from build123d import *

# Parameters (mm, degrees)
SKETCH1_W           = 20
SKETCH1_H           = 20
SKETCH1_W_2         = 11.2
SKETCH1_H_2         = 11.2
BOSS_EXTRUDE1_DEPTH = 200
SKETCH2_R           = 1.45
CUT_EXTRUDE1_DEPTH  = 202.990098767
FILLET3_SIZE        = 5
FILLET4_SIZE        = 10
SKETCH4_R           = 2.25
CUT_EXTRUDE3_DEPTH  = 202.990098886
FILLET6_R           = 1
SKETCH5_W           = 3
SKETCH5_H           = 20
CUT_EXTRUDE4_DEPTH  = 10
FILLET7_START       = 8.5
FILLET7_DEPTH       = 3
SKETCH7_R           = 0.5
CUT_EXTRUDE6_DEPTH  = 5
SKETCH8_W           = 10
SKETCH8_H           = 2.5
BOSS_EXTRUDE2_DEPTH = 10
FILLET8_R           = 5


with BuildPart() as part:
    # Sketch1 → Boss-Extrude1 (new body)
    with BuildSketch(Plane(origin=(0, 0, 0), x_dir=(1, 0, 0), z_dir=(0, 1, 0))):
        with Locations((10, -10)):
            Rectangle(SKETCH1_W, SKETCH1_H)
        with Locations((10, -10)):
            Rectangle(SKETCH1_W_2, SKETCH1_H_2, mode=Mode.SUBTRACT)
    extrude(amount=BOSS_EXTRUDE1_DEPTH)

    # Sketch2 → Cut-Extrude1 (cut, through all)
    with BuildSketch(Plane.ZY):
        with Locations((8.5, 195)):
            Circle(SKETCH2_R)
    extrude(amount=-CUT_EXTRUDE1_DEPTH, mode=Mode.SUBTRACT)

    # Fillet3
    # a fillet whose section is not a circle: 5 mm, written as the material it adds along each edge
    with BuildSketch(Plane(origin=(4.4, 0, 15.6), x_dir=(1, 0, 0), z_dir=(0, 1, 0))) as fillet3_piece_1:
        with BuildLine():
            Bezier((FILLET3_SIZE, 0), (0, 0), (0, FILLET3_SIZE), weights=[1, 0.052631579, 1])
            Line((0, FILLET3_SIZE), (0, 0))
            Line((0, 0), (FILLET3_SIZE, 0))
        make_face()
    extrude(amount=200)
    with BuildSketch(Plane(origin=(15.6, 0, 15.6), x_dir=(-1, 0, 0), z_dir=(0, 1, 0))) as fillet3_piece_2:
        with BuildLine():
            Bezier((FILLET3_SIZE, 0), (0, 0), (0, -FILLET3_SIZE), weights=[1, 0.052631579, 1])
            Line((0, -FILLET3_SIZE), (0, 0))
            Line((0, 0), (FILLET3_SIZE, 0))
        make_face()
    extrude(amount=200)

    # Fillet4
    # a fillet whose section is not a circle: 10 mm, written as the material it takes off along each edge
    with BuildSketch(Plane(origin=(0, -25, 20), x_dir=(0, 0, -1), z_dir=(0, 1, 0)), Plane(origin=(20, -25, 20), x_dir=(-1, 0, 0), z_dir=(0, 1, 0))) as fillet4_piece_1:
        with BuildLine():
            Bezier((FILLET4_SIZE, 0), (0, 0), (0, -FILLET4_SIZE), weights=[1, 0.052631579, 1])
            Line((0, -FILLET4_SIZE), (0, 0))
            Line((0, 0), (FILLET4_SIZE, 0))
        make_face()
    extrude(amount=250, mode=Mode.SUBTRACT)

    # Sketch4 → Cut-Extrude3 (cut, through all)
    with BuildSketch(Plane(origin=(0, 200, 0), x_dir=(1, 0, 0), z_dir=(0, 1, 0))):
        with Locations((10, -20)):
            Circle(SKETCH4_R)
    extrude(amount=-CUT_EXTRUDE3_DEPTH, mode=Mode.SUBTRACT)

    # Fillet6
    fillet6_edges = [part.edges().sort_by_distance(p)[0] for p in [
        (11.759792875, 100, 18.597991071),
        (8.240207125, 100, 18.597991071),
    ]]
    fillet(fillet6_edges, radius=FILLET6_R)

    # Sketch5 → Cut-Extrude4 (cut)
    with BuildSketch(Plane(origin=(0, 0, 0), x_dir=(-1, 0, 0), z_dir=(0, 0, -1))):
        with Locations((-10, 190)):
            Rectangle(SKETCH5_W, SKETCH5_H)
    extrude(amount=-CUT_EXTRUDE4_DEPTH, mode=Mode.SUBTRACT)

    # Fillet7: read off the stored shape, not the designer's step
    # Fillet7 outline → Fillet7 (cut)
    with BuildSketch(Plane.YZ.offset(FILLET7_START)):
        with BuildLine():
            Line((180, 0), (180, 2))
            add(Edge.make_bspline(
                [(180, 2), (180, 0), (178, 0)],
                knots=[0, 0, 0, 1, 1, 1], degree=2, weights=[1, 0.052631579, 1]))
            Line((178, 0), (180, 0))
        make_face()
    extrude(amount=FILLET7_DEPTH, mode=Mode.SUBTRACT)

    # Sketch7 → Cut-Extrude6 (cut)
    with BuildSketch(Plane(origin=(0, 0, 0), x_dir=(-1, 0, 0), z_dir=(0, -1, 0))):
        with Locations(Location((-10, -16.7, 0), (0, 0, 90))):
            Circle(SKETCH7_R)
    extrude(amount=-CUT_EXTRUDE6_DEPTH, mode=Mode.SUBTRACT)

    # Sketch8 → Boss-Extrude2 (add)
    with BuildSketch(Plane.ZY):
        with Locations((5, 13.25)):
            Rectangle(SKETCH8_W, SKETCH8_H)
    extrude(amount=BOSS_EXTRUDE2_DEPTH)

    # Fillet8
    fillet8_edges = [part.edges().sort_by_distance(p)[0] for p in [
        (0, 12, 5),
    ]]
    fillet(fillet8_edges, radius=FILLET8_R)


solid = part.part
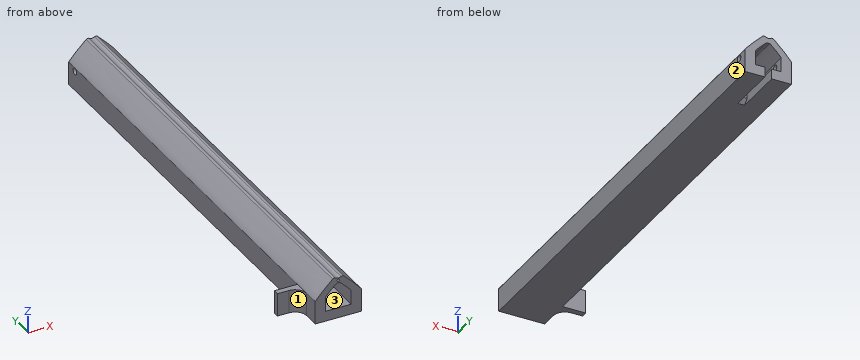
Work out the finished part from the listing and answer in its coordinate system (mm). Face numbers are marked on the shaded views. Coordinates: 2 decimals unless noted, no trailing zeros. Use one line per item in the form item = value. Start each with the question number.
1. Straight lines are drawn through the part: probe 1 along Y at (x, z) = (17.5, 8.5); probe 2 along X at (y, z) = (92, 7.25); probe 3 along Z at (x, y) = (16, 195). For each, find the intervals that lie inside material, in ascending order. Write a range as from..to.
2. Each of these flat-tipped pins is pushed along its axis until it touches: P1, Ø5, axis at x = 2.5, y = 29.5, coming from the +Z side; P2, Ø5, axis at x = 5.5, y = 34.5, coming from the +Z side; P3, Ø1.7, axis at y = 195, z = 8.5, coming from the +X side; P4, Ø8, axis at y = 149.5, z = 14.5, coming from the -X side. Where does it stop, or does it pass through?
3. The mould has two halves that part along X. Classify the marked faces 1, 2 and 3: released by +X, released by -X, zero draft, split by the parting line, or undercut.
Evaluation:
q1.probe_1 = 0..193.55, 196.45..200
q1.probe_2 = 0..4.4, 15.6..20
q1.probe_3 = 0..7.05, 9.95..14.49
q2.P1 = 15.5
q2.P2 = 18.22
q2.P3 = through
q2.P4 = 0.32
q3.face_1 = released by -X
q3.face_2 = released by +X
q3.face_3 = undercut
